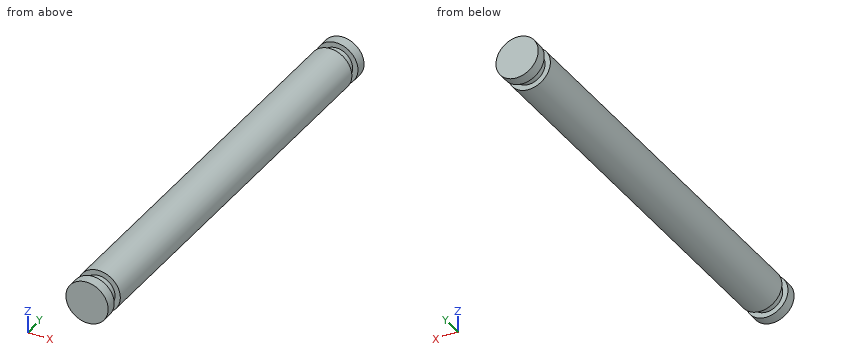
```python
from build123d import *

# Parameters (mm, degrees)
F0_R     = 2
F1_DEPTH = 42
F2_W     = 1
F2_H     = 4.527544
F2_H_2   = 5.616845


with BuildPart() as f1:
    # F0 (on Front) → F1 (new body)
    with BuildSketch(Plane.XZ):
        Circle(F0_R)
    extrude(amount=F1_DEPTH)

    # F2 (on Right) → F3 (revolve, cut)
    with BuildSketch(Plane.YZ):
        with Locations((-40.5, 3.763772)):
            Rectangle(F2_W, F2_H)
        with Locations((-1.5, 4.308422)):
            Rectangle(F2_W, F2_H_2)
    revolve(axis=Axis((0, 0, 0), (0, 1, 0)), mode=Mode.SUBTRACT)


solid = f1.part
```
Could you check a few things on this model? Use its own coordinates, in mm. Round coordinates to 2 decimals unless told otherwise and drop trailing zeros. Write each loop counter-clockwise with the first axis right and the second up, starting at its lowest first coordinate (ties: lowest second). Pieces come first, ordered by that corner, then holes. Notation, with made-up numbers: M 12.5,72 L 63.5,72 A19 ccw 63.5,89 Z; hole C -10.5,78.5 d1. An arc over 180 degrees is marked long. Answer in a Markdown table with one row per item. Add a question column.
Q1. Will this pin go through, and if not, where does the flat tip stop? pin 1 Ø2 at (x, y) = (1, -5.5) entering from -Z.
Q2. Imagine slicing it at C-C (y = -19). Please give me the cut outline in (x, z).
Q3. Imagine slicing it at A-A (z = -1.05). Please give me the cut outline in (x, y).
Q4. Imagine slicing it at B-B (x = -0.95). Please give me the cut outline in (y, z).
Q5. If I drill on line 1 (Y direction, x = 1.25, z = -1.3); line 2 (X direction, y = -6.5, z = -0.1); line 3 (Z direction, x = -0.15, y = -7.5), over which ranges is the centre line in solid material (lowest first)? Write a range as from..to.
Values:
| question | item | result |
|---|---|---|
| 1 | pin 1 | z = -2 |
| 2 | outline | C 0,0 d4 |
| 3 | outline | M -1.7,-42 L 1.7,-42 L 1.7,-41 L 1.07,-41 L 1.07,-40 L 1.7,-40 L 1.7,-2 L 1.07,-2 L 1.07,-1 L 1.7,-1 L 1.7,0 L -1.7,0 L -1.7,-1 L -1.07,-1 L -1.07,-2 L -1.7,-2 L -1.7,-40 L -1.07,-40 L -1.07,-41 L -1.7,-41 Z |
| 4 | outline | M -42,-1.76 L -41,-1.76 L -41,-1.16 L -40,-1.16 L -40,-1.76 L -2,-1.76 L -2,-1.16 L -1,-1.16 L -1,-1.76 L 0,-1.76 L 0,1.76 L -1,1.76 L -1,1.16 L -2,1.16 L -2,1.76 L -40,1.76 L -40,1.16 L -41,1.16 L -41,1.76 L -42,1.76 Z |
| 5 | line 1 | -42..-41, -40..-2, -1..0 |
| 5 | line 2 | -2..2 |
| 5 | line 3 | -1.99..1.99 |
